Autodesk Inventor part; units mm, degrees
ref_plane "YZ Plane" through (0, 0, 0) normal (1, 0, 0) x (0, 1, 0)
ref_plane "XZ Plane" through (0, 0, 0) normal (0, 1, 0) x (-1, 0, 0)
ref_plane "XY Plane" through (0, 0, 0) normal (0, 0, 1) x (1, 0, 0)
sketch "Sketch1" plane through (0, 0, 0) normal (0, 0, 1) x (1, 0, 0)
  line L0 (0, 277.6336) -> (196.3166, 196.3166) construction
  line L1 (196.3166, 196.3166) -> (277.6336, 0) construction
  line L2 (277.6336, 0) -> (196.3166, -196.3166) construction
  line L3 (196.3166, -196.3166) -> (0, -277.6336) construction
  line L4 (0, -277.6336) -> (-196.3166, -196.3166) construction
  line L5 (-196.3166, -196.3166) -> (-277.6336, 0) construction
  line L6 (-277.6336, 0) -> (-196.3166, 196.3166) construction
  line L7 (-196.3166, 196.3166) -> (0, 277.6336)
  line L8 (-196.3166, 196.3166) -> (0, 277.6336)
  line L9 (-461.2666, 773.8898) -> (-221.0579, 873.3874)
  line L10 (-98.1583, 236.9751) -> (-341.1623, 823.6386) construction
  line L11 (-221.0579, 873.3874) -> (0, 873.3874)
  line L12 (0, 873.3874) -> (0, 277.6336)
  line L13 (-461.2666, 773.8898) -> (-617.5782, 617.5782)
  line L14 (-617.5782, 617.5782) -> (-196.3166, 196.3166)
  point P0 (0, 0)
  point P1 (0, 0)
  dimension "d0" = 513
  dimension "d2" = 260
  dimension "d3" = 635
extrude "Extrusion1" add sketch "Sketch1" along normal mid plane 8
sketch "Sketch2" plane through (0, 0, 4) normal (0, 0, 1) x (1, 0, 0)
  line L0 (-221.0579, 873.3874) -> (-461.2666, 773.8898)
  line L1 (-461.2666, 773.8898) -> (-617.5782, 617.5782)
  line L2 (-236.3886, 531.4957) -> (-415.0608, 457.4872)
  line L3 (-196.3166, 196.3166) -> (0, 277.6336)
  line L4 (-98.1583, 236.9751) -> (-341.1623, 823.6386) construction
  line L5 (-617.5782, 617.5782) -> (-196.3166, 196.3166)
  line L6 (-415.0608, 457.4872) -> (-575.1518, 617.5782)
  line L7 (-575.1518, 617.5782) -> (-444.273, 748.457)
  line L8 (-444.273, 748.457) -> (-343.54, 790.182)
  line L9 (-236.3886, 531.4957) -> (-343.54, 790.182)
  line L10 (-208.6722, 542.9762) -> (-30, 616.9847)
  line L11 (-30, 616.9847) -> (-30, 843.3874)
  line L12 (-30, 843.3874) -> (-215.0906, 843.3874)
  line L13 (-215.0906, 843.3874) -> (-315.8236, 801.6625)
  line L14 (-208.6722, 542.9762) -> (-315.8236, 801.6625)
  line L15 (0, 277.6336) -> (0, 873.3874)
  line L16 (-415.0608, 457.4872) -> (-30, 616.9847) construction
  line L17 (-392.0998, 434.5262) -> (-30, 584.5129)
  line L18 (-189.2776, 231.704) -> (-30, 297.679)
  line L19 (-30, 297.679) -> (-30, 584.5129)
  line L20 (-189.2776, 231.704) -> (-392.0998, 434.5262)
  point P0 (0, 0)
  dimension "d11" = 30
  dimension "d12" = 280
  dimension "d13" = 30
  dimension "d14" = 30
  dimension "d15" = 15
  dimension "d21" = 30
  dimension "d22" = 30
  dimension "d23" = 30
  dimension "d24" = 30
extrude "Extrusion2" cut sketch "Sketch2" against normal up to surface (8 mm away)
fillet "Fillet1" radius 10 12 edges at (-575.1518, 617.5782, 0) (-343.54, 790.182, 0) (-236.3886, 531.4957, 0) (-415.0608, 457.4872, 0) (-315.8236, 801.6625, 0) (-30, 843.3874, 0) (-30, 616.9847, 0) (-208.6722, 542.9762, 0) (-392.0998, 434.5262, 0) (-30, 584.5129, 0) (-30, 297.679, 0) (-189.2776, 231.704, 0)
sketch "Sketch4" plane through (0, 0, 4) normal (0, 0, 1) x (1, 0, 0)
  line L0 (-221.0579, 873.3874) -> (-461.2666, 773.8898)
  line L1 (0, 873.3874) -> (-221.0579, 873.3874)
  line L2 (-461.2666, 773.8898) -> (-617.5782, 617.5782)
  line L3 (-617.5782, 617.5782) -> (-196.3166, 196.3166)
  line L4 (-196.3166, 196.3166) -> (0, 277.6336)
  line L5 (0, 277.6336) -> (0, 873.3874)
  line L6 (-458.4343, 769.651) -> (-220.0634, 868.3874)
  line L7 (-220.0634, 868.3874) -> (-5, 868.3874)
  line L8 (-5, 868.3874) -> (-5, 280.9745)
  line L9 (-5, 280.9745) -> (-195.1434, 202.2145)
  line L10 (-195.1434, 202.2145) -> (-610.5071, 617.5782)
  line L11 (-610.5071, 617.5782) -> (-458.4343, 769.651)
  line L12 (-218.4721, 860.3874) -> (-453.9027, 762.8689)
  line L13 (-453.9027, 762.8689) -> (-599.1934, 617.5782)
  line L14 (-599.1934, 617.5782) -> (-193.2664, 211.6511)
  line L15 (-193.2664, 211.6511) -> (-13, 286.3199)
  line L16 (-13, 286.3199) -> (-13, 860.3874)
  line L17 (-13, 860.3874) -> (-218.4721, 860.3874)
  point P0 (0, 0)
  dimension "d26" = 5
  dimension "d27" = 8
extrude "Extrusion3" cut sketch "Sketch4" against normal blind 3 contours L6 L7 L8 L9 L10 L11
fillet "Fillet3" radius 16 2 edges at (-220.0634, 868.3874, 2.5) (-458.4343, 769.651, 2.5)
fillet "Fillet4" radius 8 2 edges at (-453.9027, 762.8689, 2.5) (-218.4721, 860.3874, 2.5)
equation "\"d0\" = Барабан_габарит_по_кассетам"
equation "\"d2\" = Кассета_длина_грани"
equation "\"d3\" = Кассета_высота"
equation "\"d11\" = d13"
equation "\"d14\" = d13"
equation "\"d15\" = 0.5 * d13"
equation "\"d21\" = d13"
equation "\"d22\" = d13"
equation "\"d23\" = d13"
equation "\"d24\" = d13"
properties part number "ДМФ 01 51 Внешняя рамка"
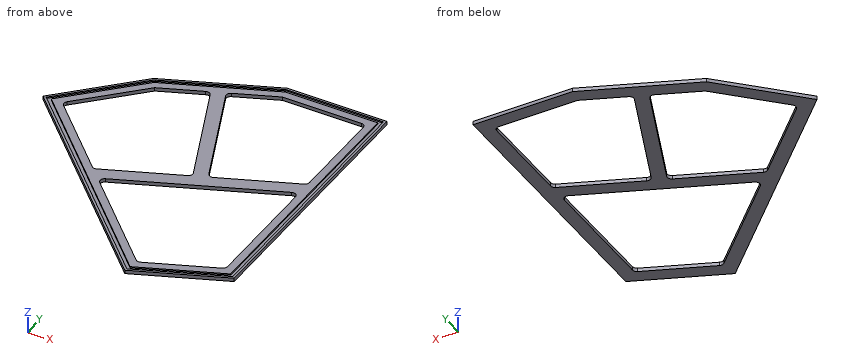
Check sheet for the modelled part. Datum: model origin and axes. Units: mm. Round coordinates to 2 decimals unless told otherwise and drop trailing zeros. Loops run counter-clockwise (first coordinate to the right, second up) from the corner with the lowest first, then second, coordinate; pieces in that order, holes last. Notation, with made-up numbers: (57.5, 48) -> (84.5, 48) arc R8 cw to (84.5, 57) -> close; hole circle Ø8 at (64.5, 42). An arc over 180 degrees is marked (long way). Put each result on its own line as item: value. Start each with the question number.
1. Section check C-C (y = 313). Enter the section's corners in (x, z), plus the area to 3 significant figures.
2. Section check B-B (x = -369). Enter the section's corners in (y, z).
3. Gauge pin test, flat ends, axial feed: pin 1 (2.5 mm diameter, centred on y = 407, z = -1, fed in from -X); pin 2 (1 mm diameter, centred on x = -98, z = -0.5, fed in from -Y); pin 3 (2.5 mm diameter, centred on x = -155, z = 2, fed in from -Y); pin 4 (2.5 mm diameter, centred on y = 498, z = 3, fed in from +X). Record the tip position at first contact, or that the pin passes through.
4. Scan lines: probe 1 along X at (y, z) = (637, 3.5); probe 2 along Y at (x, z) = (-220, -2.25); probe 3 along X at (y, z) = (660, 1.5). Record each from-to range of solid material in increasing order.
5. Section check A-A (z = -0.5). Give the number of separate pieces and of enclosed holes in the cut face, plus the area to 3 significant figures.
6. Section check D-D (x = -434.5). Enter the section's corners in (y, z), plus the area to 3 significant figures.
Findings:
1. outline: (-313, -4) -> (-270.57, -4) -> (-270.57, 4) -> (-294.62, 4) -> (-294.62, 1) -> (-305.93, 1) -> (-305.93, 4) -> (-313, 4) -> close; (-30, -4) -> (0, -4) -> (0, 4) -> (-5, 4) -> (-5, 1) -> (-13, 1) -> (-13, 4) -> (-30, 4) -> close
1. area: 521 mm^2
2. outline: (369, -4) -> (411.43, -4) -> (411.43, 4) -> (387.38, 4) -> (387.38, 1) -> (376.07, 1) -> (376.07, 4) -> (369, 4) -> close; (444.09, -4) -> (476.57, -4) -> (476.57, 4) -> (444.09, 4) -> close; (779.64, -4) -> (812.11, -4) -> (812.11, 4) -> (806.7, 4) -> (806.7, 1) -> (798.04, 1) -> (798.04, 4) -> (779.64, 4) -> close
3. pin 1: stops at x = -408.25
3. pin 2: stops at y = 236.83
3. pin 3: stops at y = 212.91
3. pin 4: stops at x = 0
4. probe 1: x = -598.16 to -591.09, -579.77 to -555.73, -280.09 to -247.62, -30 to -13, -5 to 0
4. probe 2: y = 220 to 262.43, 505.81 to 570.32, 841.35 to 873.39
4. probe 3: x = -575.16 to -568.09, -556.77 to -532.73, -289.62 to -257.15, -30 to -13, -5 to 0
5. separate pieces: 1
5. enclosed holes: 3
5. area: 80,600 mm^2
6. outline: (434.5, -4) -> (476.93, -4) -> (476.93, 4) -> (452.88, 4) -> (452.88, 1) -> (441.57, 1) -> (441.57, 4) -> (434.5, 4) -> close; (752.51, -4) -> (784.98, -4) -> (784.98, 4) -> (779.56, 4) -> (779.56, 1) -> (770.91, 1) -> (770.91, 4) -> (752.51, 4) -> close
6. area: 539 mm^2
